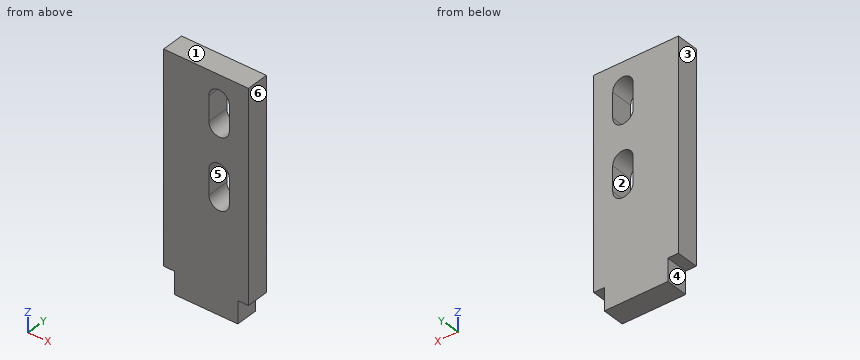
from build123d import *

# Parameters (mm, degrees)
BOSS_EXTRUDE1_DEPTH = 3.175


with BuildPart() as part:
    # Sketch1 → Boss-Extrude1 (new body)
    with BuildSketch(Plane(origin=(0, 0, 0), x_dir=(1, 0, 0), z_dir=(0, 1, 0))):
        Polygon((-32.35, -10.25), (-20.35, -10.25), (-20.35, 19.25), (-21.85, 19.25), (-21.85, 22.425), (-30.85, 22.425), (-30.85, 19.25), (-32.35, 19.25), align=None)
        with BuildLine():
            Line((-25.95, -6.75), (-25.95, -3.25))
            ThreePointArc((-25.95, -3.25), (-24.5, -1.8), (-23.05, -3.25))
            Line((-23.05, -3.25), (-23.05, -6.75))
            ThreePointArc((-23.05, -6.75), (-24.5, -8.2), (-25.95, -6.75))
        make_face(mode=Mode.SUBTRACT)
        with BuildLine():
            Line((-25.95, 3.25), (-25.95, 6.75))
            ThreePointArc((-25.95, 6.75), (-24.5, 8.2), (-23.05, 6.75))
            Line((-23.05, 6.75), (-23.05, 3.25))
            ThreePointArc((-23.05, 3.25), (-24.5, 1.8), (-25.95, 3.25))
        make_face(mode=Mode.SUBTRACT)
    extrude(amount=BOSS_EXTRUDE1_DEPTH)


solid = part.part
Verification items for the finished model (mm, model axes). Face numbers are marked on the shaded views. A direction names the side the tool comes from. Coordinates: 2 decimals unless noted, no trailing zeros. Order: outer loops, then holes, each group sorted by start corner. A loop starts at its lowest first (then second) coordinate and runs counter-clockwise, first axis right, second up. Notation, with made-up numbers: (72.5, 58) -> (127.5, 58) arc R17 cw to (127.5, 77) -> close; hole circle Ø8 at (-21, -4). An arc over 180 degrees is marked (long way). Put each result on its own line as item: value. Start each with the question number.
1. Go/stop test with flat-tipped pins: pin 1 Ø1 at (y, z) = (1, -20.5) entering from -X; pin 2 Ø1 at (y, z) = (1, -20.5) entering from +X. Record where each tip stops, or that it passes through.
2. Cross-section at B-B, the plane y = 1.5. Record the boundary of the cut face in (x, z) (3 decimals), then the cut area to 3 significant figures.
3. Mould release check, pull along X, two halves, no side actions. Record for the marked faces 1, 2 and 3: released by +X, released by -X, zero draft, split by the parting line, or undercut.
4. Cross-section at C-C, the plane x = -21. Record the boundary of the cut face in (y, z) (3 decimals).
5. Cross-section at A-A, the plane x = -24.5. Record the boundary of the cut face in (y, z) (3 decimals).
6. Access from +Z, -Z, +X, -X, +Y, -Y to the whole of each face (thin tool, end or side, straight path). Record for the marked faces 4, 5 and 6.
7. Material ranges on L1, parallel to X at y = 2.45, z = 4; L2, parallel to Z at x = -31.25, y = 1.5; L3, parallel to Z at x = -25.25, y = 1.25 (3 decimals), recorded low to high. Write a range as [from, to].
Computed:
1. pin 1: x = -30.85
1. pin 2: x = -21.85
2. outline: (-32.35, -19.25) -> (-30.85, -19.25) -> (-30.85, -22.425) -> (-21.85, -22.425) -> (-21.85, -19.25) -> (-20.35, -19.25) -> (-20.35, 10.25) -> (-32.35, 10.25) -> close; hole (-25.95, -6.75) arc R1.45 ccw to (-23.05, -6.75) -> (-23.05, -3.25) arc R1.45 ccw to (-25.95, -3.25) -> close; hole (-25.95, 3.25) arc R1.45 ccw to (-23.05, 3.25) -> (-23.05, 6.75) arc R1.45 ccw to (-25.95, 6.75) -> close
2. area: 349 mm2
3. face 1: zero draft
3. face 2: undercut
3. face 3: released by -X
4. outline: (0, -19.25) -> (3.175, -19.25) -> (3.175, 10.25) -> (0, 10.25) -> close
5. outline: (0, -22.425) -> (3.175, -22.425) -> (3.175, -8.2) -> (0, -8.2) -> close; (0, -1.8) -> (3.175, -1.8) -> (3.175, 1.8) -> (0, 1.8) -> close; (0, 8.2) -> (3.175, 8.2) -> (3.175, 10.25) -> (0, 10.25) -> close
6. face 4: -Z, -X, +Y, -Y
6. face 5: +Y, -Y
6. face 6: +Z, -Z, +X, +Y, -Y
7. L1: [-32.35, -25.95], [-23.05, -20.35]
7. L2: [-19.25, 10.25]
7. L3: [-22.425, -7.991], [-2.009, 2.009], [7.991, 10.25]
